from build123d import *

# Parameters (mm, degrees)
SKETCH2_W           = 16
SKETCH2_H           = 16
BOSS_EXTRUDE1_DEPTH = 16
SKETCH3_OUTSIDE_W   = 81.914
SKETCH3_OUTSIDE_H   = 81.914
SKETCH3_OUTSIDE_R   = 8
CUT_EXTRUDE1_DEPTH  = 10
CUT_EXTRUDE1_DRAFT  = -60
SKETCH4_OUTSIDE_W   = 81.914
SKETCH4_OUTSIDE_H   = 81.914
SKETCH4_OUTSIDE_R   = 8
CUT_EXTRUDE2_DEPTH  = 10
CUT_EXTRUDE2_DRAFT  = -60


with BuildPart() as part:
    # Sketch1 → Revolve1 (revolve)
    with BuildSketch(Plane.XY):
        Polygon((0, 0), (-7, 0), (-7, 10), (-8, 10), (-8, 55), (-13.5, 55), (-13.5, 58), (-8, 58), (-8, 67), (0, 67), align=None)
    revolve(axis=Axis((0, 67, 0), (0, -1, 0)))

    # Sketch2 → Boss-Extrude1 (add)
    with BuildSketch(Plane(origin=(0, 67, 0), x_dir=(1, 0, 0), z_dir=(0, 1, 0))):
        Rectangle(SKETCH2_W, SKETCH2_H)
    extrude(amount=BOSS_EXTRUDE1_DEPTH)


with BuildPart() as cut_extrude1_tool:
    # Sketch3 outside → Cut-Extrude1 (with draft: the straight prism first)
    with BuildSketch(Plane(origin=(0, 83, 0), x_dir=(1, 0, 0), z_dir=(0, 1, 0))):
        Rectangle(SKETCH3_OUTSIDE_W, SKETCH3_OUTSIDE_H)
        with Locations(Location((0, 0, 0), (0, 0, 180))):
            Circle(SKETCH3_OUTSIDE_R, mode=Mode.SUBTRACT)
    extrude(amount=-CUT_EXTRUDE1_DEPTH)
    # Cut-Extrude1: the draft: its side faces are tilted about the plane it starts from
    cut_extrude1_sides = [cut_extrude1_tool.faces().sort_by_distance(p)[0] for p in [
        (0, 78, 40.957),
        (40.957, 78, 0),
        (0, 78, -40.957),
        (-40.957, 78, 0),
        (8, 78, 0),
    ]]
    draft(cut_extrude1_sides, Plane(origin=(0, 83, 0), x_dir=(1, 0, 0), z_dir=(0, 1, 0)), CUT_EXTRUDE1_DRAFT)


with BuildPart() as part_1:
    add(part.part)

    # Cut-Extrude1: cut by cut_extrude1_tool
    add(cut_extrude1_tool.part, mode=Mode.SUBTRACT)


with BuildPart() as cut_extrude2_tool:
    # Sketch4 outside → Cut-Extrude2 (with draft: the straight prism first)
    with BuildSketch(Plane.XZ.offset(-67)):
        Rectangle(SKETCH4_OUTSIDE_W, SKETCH4_OUTSIDE_H)
        with Locations(Location((0, 0, 0), (0, 0, 180))):
            Circle(SKETCH4_OUTSIDE_R, mode=Mode.SUBTRACT)
    extrude(amount=-CUT_EXTRUDE2_DEPTH)
    # Cut-Extrude2: the draft: its side faces are tilted about the plane it starts from
    cut_extrude2_sides = [cut_extrude2_tool.faces().sort_by_distance(p)[0] for p in [
        (0, 72, -40.957),
        (40.957, 72, 0),
        (0, 72, 40.957),
        (-40.957, 72, 0),
        (8, 72, 0),
    ]]
    draft(cut_extrude2_sides, Plane.XZ.offset(-67), CUT_EXTRUDE2_DRAFT)


with BuildPart() as part_2:
    add(part_1.part)

    # Cut-Extrude2: cut by cut_extrude2_tool
    add(cut_extrude2_tool.part, mode=Mode.SUBTRACT)


solid = part_2.part
Verification items for the finished model (mm, model axes). A direction names the side the tool comes from. Give positions to 0.01 mm unless a question says otherwise; leave off trailing zeros. Order: outer loops, then holes, each group sorted by start corner. A loop starts at its lowest first (then second) coordinate and runs counter-clockwise, first axis right, second up. Notation, with made-up numbers: M 48,7 L 60,7 A21 ccw 60,14 Z; hole C 65,48 d2. An arc over 180 degrees is marked long. Answer as a JSON object with one key per item and string values. Group by question number.
1) Mould release check, pull along Y, two halves, no side actions. Record for faces 4 (the face through (4, 10, 6)), 5 (the face through (-6.193, 67.456, 6.238)), 6 (the face through (0, 83, 0)), 7 (the face through (1.73, 32.82, 7.81)): released by +Y, released by -Y, zero draft, split by the parting line, or undercut.
2) Cross-section at B-B (z = 10). Enter the section's corners in (x, y), then the cut area to 3 significant figures.
3) Depth check by flat-ended pin: pin 1 Ø13 at (x, y) = (0, 74.5) entering from -Z; pin 2 Ø2 at (y, z) = (72, 3.5) entering from +X; pin 3 Ø6 at (x, z) = (9.5, 10.5) entering from +Y. Enter the tip coordinate at first touch or a pass-through.
4) Access from +Z, -Z, +X, -X, +Y, -Y to the whole of each face (thin tool, end or side, straight path). Record for faces 1 (the face through (0, 75, -8)), 2 (the face through (8, 75, 0)), 3 (the face through (-8, 75, 0)).
5) Cross-section at A-A (y = 14). Enter the section's corners in (x, z), then the cut area to 3 significant figures.
6) Scan lines: line 1 along Z through (x, y) = (-1, 71.5); line 2 along Y through (x, z) = (-5, -10.75); line 3 along Y through (x, z) = (4, -7). Record each from-to range of solid material in increasing order. Write a range as [from, to].
7) Cross-section at C-C (x = -8.75). Enter the section's corners in (y, z).
Result sheet:
{
 "1": {"face 4": "released by -Y", "face 5": "undercut", "face 6": "released by +Y", "face 7": "zero draft"},
 "2": {"outline": "M -9.07,55 L 9.07,55 L 9.07,58 L -9.07,58 Z", "area": "54.4 mm2"},
 "3": {"pin 1": "stops at z = -8", "pin 2": "stops at x = 8", "pin 3": "stops at y = 81.15"},
 "4": {"face 1": "-Z, +X, -X, +Y", "face 2": "+Z, -Z, +X, +Y", "face 3": "+Z, -Z, -X, +Y"},
 "5": {"outline": "C 0,0 d16", "area": "201 mm2"},
 "6": {"line 1": "z = [-8, 8]", "line 2": "y = [55, 58]", "line 3": "y = [55, 58], [67.04, 82.96]"},
 "7": {"outline": "M 55,-10.28 L 58,-10.28 L 58,10.28 L 55,10.28 Z"}
}
